Design review of the part built by this model. Coordinates are the model's own, in mm. Face numbers are marked on the shaded views. A direction names the side the tool comes from. Round coordinates to 2 decimals unless told otherwise and drop trailing zeros. Loops run counter-clockwise (first coordinate to the right, second up) from the corner with the lowest first, then second, coordinate; pieces in that order, holes last. Notation, with made-up numbers: (89.5, -2) - (125.5, -2) arc R9 ccw to (125.5, 15) - close; hole circle Ø4 at (-1, 87.5). An arc over 180 degrees is marked (long way). Use one line per item in the form item = value. Start each with the question number.
(1) We need section C-C, the plane z = -1.2. Give the number of separate pieces and of enclosed holes in the cut face, then the cut area to 3 significant figures.
(2) We need section D-D, the plane x = -6. Write out the cut boundary in (y, z), then the cut area to 3 significant figures.
(3) We need section A-A, the plane y = -1.5. Write out the cut boundary in (x, z).
(4) The part is to be moulded in two halves that separate along Y. For the marked faces 5, 6 and 7, say which applies: released by +Y, released by -Y, zero draft, split by the parting line, or undercut.
(5) For pin 1 (1.2 mm diameter, centred on y = 7, z = -2.5, fed in from -X); pin 2 (2 mm diameter, centred on y = -3, z = -3, fed in from -X); pin 3 (3.5 mm diameter, centred on x = -9.65, y = 3.47, fed in from -Z), all flat-tipped, find the tip position at first contact; note any pin that passes through.
(6) We need section B-B, the plane z = -4.55. Write out the cut boundary in (x, y), then the cut area to 3 significant figures.
(7) Wall thickness on probe 1 along X at (y, z) = (0.5, -0.65); probe 2 along X at (y, z) = (-3, -1.6); probe 3 along Y at (x, z) = (3.5, -4.15): over which ranges is each line inside the solid? List them lowest first. Write a range as [from, to].
(8) Machinability: for the marked faces 1, 2, 3 and 4, which of the approach directions +Z, -Z, +X, -X, +Y, -Y give a long, thin tool a straight path to every point of the face, cutting with its end or side? Answer none if there is none.
from build123d import *

# Parameters (mm, degrees)
BOSS_EXTRUDE1_DEPTH = 5
SKETCH2_W           = 3.175
SKETCH2_H           = 4
BOSS_EXTRUDE2_DEPTH = 7
SKETCH5_R           = 1.5875
CUT_EXTRUDE3_DEPTH  = 3.175
SKETCH6_W           = 2
SKETCH6_H           = 3
CUT_EXTRUDE4_DEPTH  = 5
SKETCH7_R           = 0.75
CUT_EXTRUDE5_DEPTH  = 1


with BuildPart() as part:
    # Sketch1 → Boss-Extrude1 (new body)
    with BuildSketch(Plane.XY):
        Polygon((-0.65091967, 7.716869785), (-3.15091967, 7.716869785), (-3.15091967, 5.466869785), (-4.65091967, 5.466869785), (-4.65091967, 1.466869785), (-3.15091967, 1.466869785), (-3.15091967, -0.783130215), (-0.65091967, -0.783130215), (-0.65091967, 0.716869785), (0.59908033, 0.716869785), (0.59908033, -4.283130215), (4.59908033, -4.283130215), (4.59908033, 0.466869785), (4.59908033, 0.716869785), (5.84908033, 0.716869785), (5.84908033, -0.783130215), (8.34908033, -0.783130215), (8.34908033, 1.466869785), (9.84908033, 1.466869785), (9.84908033, 5.466869785), (8.34908033, 5.466869785), (8.34908033, 7.716869785), (5.84908033, 7.716869785), (5.84908033, 6.216869785), (-0.65091967, 6.216869785), align=None)
    extrude(amount=-BOSS_EXTRUDE1_DEPTH)

    # Sketch2 → Boss-Extrude2 (add)
    with BuildSketch(Plane.ZY.offset(4.65091967)):
        with Locations((-2.5, 3.466869785)):
            Rectangle(SKETCH2_W, SKETCH2_H)
    extrude(amount=BOSS_EXTRUDE2_DEPTH)

    # Sketch5 → Cut-Extrude3 (cut)
    with BuildSketch(Plane.XY.offset(-0.9125)):
        with BuildLine():
            ThreePointArc((-11.65091967, 3.466869785), (-11.065133233, 4.881083347), (-9.65091967, 5.466869785))
            Line((-9.65091967, 5.466869785), (-11.65091967, 5.466869785))
            Line((-11.65091967, 5.466869785), (-11.65091967, 3.466869785))
        make_face()
        with BuildLine():
            ThreePointArc((-9.65091967, 1.466869785), (-11.065133233, 2.052656222), (-11.65091967, 3.466869785))
            Line((-11.65091967, 3.466869785), (-11.65091967, 1.466869785))
            Line((-11.65091967, 1.466869785), (-9.65091967, 1.466869785))
        make_face()
        with Locations((-9.65091967, 3.466869785)):
            Circle(SKETCH5_R)
    extrude(amount=-CUT_EXTRUDE3_DEPTH, mode=Mode.SUBTRACT)

    # Sketch6 → Cut-Extrude4 (cut)
    with BuildSketch(Plane.XY):
        with Locations((2.59908033, -1.783130215)):
            Rectangle(SKETCH6_W, SKETCH6_H)
    extrude(amount=-CUT_EXTRUDE4_DEPTH, mode=Mode.SUBTRACT)

    # Sketch7 → Cut-Extrude5 (cut)
    with BuildSketch(Plane.XZ.offset(4.283130215)):
        with Locations((2.59908033, -2.5)):
            Circle(SKETCH7_R)
    extrude(amount=-CUT_EXTRUDE5_DEPTH, mode=Mode.SUBTRACT)


solid = part.part
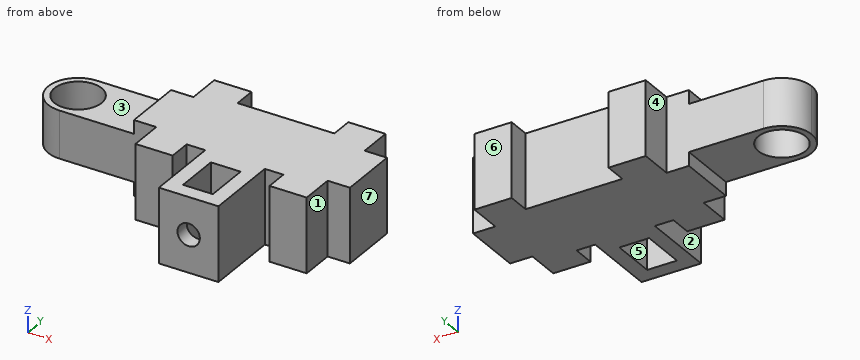
Data:
q1.separate_pieces = 1
q1.enclosed_holes = 2
q1.area = 123 mm^2
q2.outline = (1.47, -4.09) - (5.47, -4.09) - (5.47, -0.91) - (1.47, -0.91) - close
q2.area = 12.7 mm^2
q3.outline = (0.6, -5) - (1.6, -5) - (1.6, 0) - (0.6, 0) - close; (3.6, -5) - (4.6, -5) - (4.6, 0) - (3.6, 0) - close
q4.face_5 = undercut
q4.face_6 = released by +Y
q4.face_7 = zero draft
q5.pin_1 = -3.15
q5.pin_2 = 0.6
q5.pin_3 = -4.09
q6.outline = (-4.65, 1.47) - (-3.15, 1.47) - (-3.15, -0.78) - (-0.65, -0.78) - (-0.65, 0.72) - (0.6, 0.72) - (0.6, -4.28) - (4.6, -4.28) - (4.6, 0.72) - (5.85, 0.72) - (5.85, -0.78) - (8.35, -0.78) - (8.35, 1.47) - (9.85, 1.47) - (9.85, 5.47) - (8.35, 5.47) - (8.35, 7.72) - (5.85, 7.72) - (5.85, 6.22) - (-0.65, 6.22) - (-0.65, 7.72) - (-3.15, 7.72) - (-3.15, 5.47) - (-4.65, 5.47) - close; hole (1.6, -3.28) - (3.6, -3.28) - (3.6, -0.28) - (1.6, -0.28) - close
q6.area = 104 mm^2
q7.probe_1 = [-3.15, -0.65], [0.6, 4.6], [5.85, 8.35]
q7.probe_2 = [0.6, 1.6], [3.6, 4.6]
q7.probe_3 = [-4.28, -3.28], [-0.28, 6.22]
q8.face_1 = +Z, -Z, +X, -Y
q8.face_2 = +Z, -Z, -Y
q8.face_3 = +Z, -X, +Y, -Y
q8.face_4 = +Z, -Z, -X, +Y
